```python
from build123d import *

# Parameters (mm, degrees)
SKETCH1_R           = 26
BOSS_EXTRUDE1_DEPTH = 90
SKETCH2_R           = 8.638646247
BOSS_EXTRUDE2_DEPTH = 5
SKETCH3_R           = 26
BOSS_EXTRUDE3_DEPTH = 15
SKETCH4_R           = 10.67473996
BOSS_EXTRUDE4_DEPTH = 5
SKETCH5_R           = 2.5
BOSS_EXTRUDE5_DEPTH = 25
FILLET1_R           = 6


with BuildPart() as part:
    # Sketch1 → Boss-Extrude1 (new body)
    with BuildSketch(Plane(origin=(0, 0, 0), x_dir=(1, 0, 0), z_dir=(0, 1, 0))):
        with Locations(Location((0, 0, 0), (0, 0, 90))):
            Circle(SKETCH1_R)
    extrude(amount=BOSS_EXTRUDE1_DEPTH)

    # Sketch2 → Boss-Extrude2 (add)
    with BuildSketch(Plane(origin=(0, 90, 0), x_dir=(1, 0, 0), z_dir=(0, 1, 0))):
        with Locations(Location((0, 0, 0), (0, 0, 270))):
            Circle(SKETCH2_R)
    extrude(amount=BOSS_EXTRUDE2_DEPTH)

    # Sketch3 → Boss-Extrude3 (add)
    with BuildSketch(Plane(origin=(0, 95, 0), x_dir=(1, 0, 0), z_dir=(0, 1, 0))):
        with Locations(Location((0, 0, 0), (0, 0, 90))):
            Circle(SKETCH3_R)
    extrude(amount=BOSS_EXTRUDE3_DEPTH)

    # Sketch4 → Boss-Extrude4 (add)
    with BuildSketch(Plane.XZ):
        with Locations(Location((0, 0, 0), (0, 0, 90))):
            Circle(SKETCH4_R)
    extrude(amount=BOSS_EXTRUDE4_DEPTH)

    # Sketch5 → Boss-Extrude5 (add)
    with BuildSketch(Plane.XZ.offset(5)):
        with Locations(Location((0, 0, 0), (0, 0, 270))):
            Circle(SKETCH5_R)
    extrude(amount=BOSS_EXTRUDE5_DEPTH)

    # Fillet1
    fillet1_edges = [part.edges().sort_by_distance(p)[0] for p in [
        (0, 110, 26),
    ]]
    fillet(fillet1_edges, radius=FILLET1_R)


solid = part.part
```
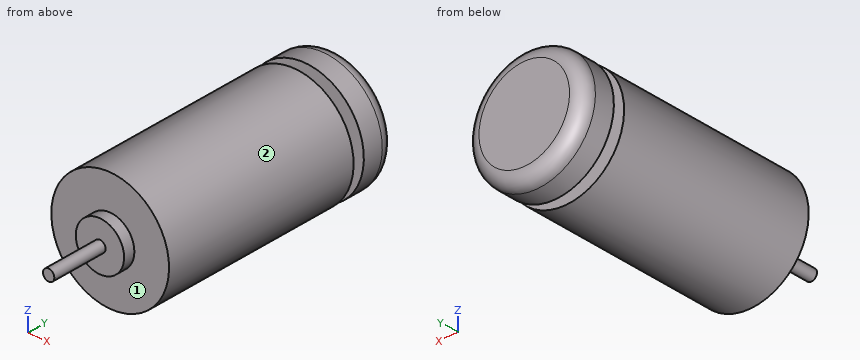
Part model, mm, in its own coordinate system. Face numbers are marked on the shaded views. A direction names the side the tool comes from. Give positions to 0.01 mm unless a question says otherwise; leave off trailing zeros. Write each loop counter-clockwise with the first axis right and the second up, starting at its lowest first coordinate (ties: lowest second). Pieces come first, ordered by that corner, then holes. Notation, with made-up numbers: M 13,19.5 L 41,19.5 A11 ccw 41,37.5 Z; hole C 46.5,62 d7. An arc over 180 degrees is marked long. Use CSV: the item, a comma, the result in double quotes.
Item 1: Slice it at A-A on z = 0. Write the cut outline in (x, y), plus the area to 3 significant figures.
Taken from the geometry:
outline,"M -26,0 L -10.67,0 L -10.67,-5 L -2.5,-5 L -2.5,-30 L 2.5,-30 L 2.5,-5 L 10.67,-5 L 10.67,0 L 26,0 L 26,90 L 8.64,90 L 8.64,95 L 26,95 L 26,104 A6 ccw 20,110 L -20,110 A6 ccw -26,104 L -26,95 L -8.64,95 L -8.64,90 L -26,90 Z"
area,"5,760 mm²"
Item 2: Slice it at C-C on y = 5.5. Write the cut outline in (x, z).
Taken from the geometry:
outline,"C 0,0 d52"
Item 3: Slice it at B-B on x = 0. Write the cut outline in (y, z), plus the area to 3 significant figures.
Taken from the geometry:
outline,"M -30,-2.5 L -5,-2.5 L -5,-10.67 L 0,-10.67 L 0,-26 L 90,-26 L 90,-8.64 L 95,-8.64 L 95,-26 L 104,-26 A6 ccw 110,-20 L 110,20 A6 ccw 104,26 L 95,26 L 95,8.64 L 90,8.64 L 90,26 L 0,26 L 0,10.67 L -5,10.67 L -5,2.5 L -30,2.5 Z"
area,"5,760 mm²"
Item 4: Which spindle directions (+Z, -Z, +X, -X, +Y, -Y) get a long thin tool onto all of the face, cutting with end or side? Do the marked faces 1 and 2. Say none if no direction does.
Taken from the geometry:
face 1,"-Y"
face 2,"+Y, -Y"
Item 5: Drill centre lines: probe 1 along Y at (x, z) = (6.5, 11.5); probe 2 along Y at (x, z) = (9.5, -1); probe 3 along Z at (x, y) = (10, 17). Where is each one in solid material? Low to high.
Taken from the geometry:
probe 1,"y = 0 to 90, 95 to 110"
probe 2,"y = -5 to 90, 95 to 110"
probe 3,"z = -24 to 24"
Item 6: Pin check, flat tips, straight feed: P1, Ø1.5, axis at y = 68, z = -9, coming from the +X side; P2, Ø6, axis at y = 13, z = -8, coming from the +X side; P3, Ø12, axis at x = 20.5, y = 39.5, coming from the +Z side; P4, Ø1, axis at x = -12, y = -2, coming from the +Z side. Stop position of each tip, or through.
Taken from the geometry:
P1,"stops at x = 24.66"
P2,"stops at x = 25.51"
P3,"stops at z = 21.58"
P4,"passes through"
